Autodesk Inventor part; units mm, degrees
ref_plane "YZ Plane" through (0, 0, 0) normal (1, 0, 0) x (0, 1, 0)
ref_plane "XZ Plane" through (0, 0, 0) normal (0, 1, 0) x (-1, 0, 0)
ref_plane "XY Plane" through (0, 0, 0) normal (0, 0, 1) x (1, 0, 0)
sketch "Sketch1" plane through (0, 0, 0) normal (0, 0, 1) x (1, 0, 0)
  line L0 (-53.34, 0) -> (53.34, 0)
  line L1 (0, -7.0485) -> (0, 42.291)
  line L2 (-38.1, 0) -> (38.1, 0)
  arc A0 (16.1925, 19.05) -> (-16.1925, 19.05) centre (0, 19.05) ccw
  line L3 (-38.1, 6.35) -> (-22.5425, 6.35)
  line L4 (22.5425, 6.35) -> (38.1, 6.35)
  line L5 (38.1, 0) -> (38.1, 6.35)
  line L6 (-38.1, 0) -> (-38.1, 6.35)
  line L7 (-16.1925, 19.05) -> (-16.1925, 12.7)
  line L8 (16.1925, 19.05) -> (16.1925, 12.7)
  arc A1 (-22.5425, 6.35) -> (-16.1925, 12.7) centre (-22.5425, 12.7) ccw
  arc A2 (16.1925, 12.7) -> (22.5425, 6.35) centre (22.5425, 12.7) ccw
  point P0 (0, 0)
  point P1 (-10.0453, 6.35)
  point P2 (10.0453, 6.35)
  dimension "d0" = 76.2
  dimension "d1" = 32.385
  dimension "d4" = 6.35
  dimension "d5" = 19.05
  dimension "d6" = 6.35
extrude "Extrusion1" add sketch "Sketch1" along normal mid plane 12.7
sketch "Sketch2" plane through (0, 0, 6.35) normal (0, 0, 1) x (1, 0, 0)
  arc A0 (16.1925, 19.05) -> (-16.1925, 19.05) centre (0, 19.05) ccw
  circle A1 centre (0, 19.05) radius 14.3129
  point P0 (0, 0)
  dimension "d9" = 28.6258
extrude "Extrusion2" cut sketch "Sketch2" against normal blind 11.1125
sketch "Sketch3" plane through (0, 19.05, -4.7625) normal (0, 0, 1) x (1, 0, 0)
  circle A0 centre (0, 0) radius 14.3129
  circle A1 centre (0, 0) radius 7.9375
  point P0 (0, -19.05)
  dimension "d14" = 15.875
extrude "Extrusion3" cut sketch "Sketch3" against normal through all contours A1
sketch "Sketch4" plane through (-38.1, 6.35, 6.35) normal (0, 1, 0) x (1, 0, 0)
  line L0 (15.5575, 12.7) -> (0, 12.7)
  arc A0 (5.3975, 9.7282) -> (5.3975, 2.9718) centre (5.3975, 6.35) ccw
  line L1 (-15.24, 6.35) -> (91.44, 6.35)
  line L2 (38.1, 15.24) -> (38.1, -2.54)
  arc A1 (10.16, 2.9718) -> (10.16, 9.7282) centre (10.16, 6.35) ccw
  line L3 (10.16, 9.7282) -> (5.3975, 9.7282)
  line L4 (10.16, 2.9718) -> (5.3975, 2.9718)
  line L5 (7.7788, 2.9718) -> (7.7788, 9.7282) construction
  point P0 (38.1, 6.35)
  point P1 (7.7788, 12.7)
  dimension "d16" = 3.3782
  dimension "d17" = 4.7625
extrude "Mount Slot" cut sketch "Sketch4" against normal through all
mirror "Mirror1" about plane through (0, 0, 0) normal (1, 0, 0) of "Mount Slot"
properties part number "side mount bearing block"
Part model, mm, in its own coordinate system. A direction names the side the tool comes from. Coordinates: 2 decimals unless noted, no trailing zeros. Loops run counter-clockwise (first coordinate to the right, second up) from the corner with the lowest first, then second, coordinate; pieces in that order, holes last. Notation, with made-up numbers: (-32.5, 58) - (-9.5, 58) arc R33 ccw to (-9.5, 97) - close; hole circle Ø6 at (87, 68.5). An arc over 180 degrees is marked (long way). Write item = value, one per line. Start each with the question number.
Item 1: Flat gauge pins, fed straight in: pin 1 Ø2 at (y, z) = (15, 3.5) entering from -X; pin 2 Ø1 at (x, z) = (21, 4) entering from +Y; pin 3 Ø7 at (y, z) = (14.5, 2) entering from +X. Where does each tip first touch, or does it go through?
Item 2: Cut at B-B, the plane x = 0. Give the cut face in (y, z), and give its area (3 significant figures).
Item 3: Cut at D-D, the plane x = -13.5. Give the cut face in (y, z), and give its area (3 significant figures).
Item 4: 3-axis set-ups, long thin cutter, end or side, ignore diameter. For faces 1 (the flat face through (6, 13, -4.762)), 2 (the flat face through (30, 6.35, -4)), 3 (the flat face through (-30, 6.35, -4)), 4 (the flat face through (-30, 3, 3.378)): which of +Z, -Z, +X, -X, +Y, -Y reach the whole face in a straight line?
Item 5: Cut at C-C, the plane y = 21. Give the cut face in (x, z).
Item 6: Cut at A-A, the plane z = 0. State how many separate pieces and enclosed holes the cut face has, and give its area (3 significant figures).
Item 7: Wall check: L1, parallel to Y at x = 0, z = 4; L2, parallel to Y at x = 0, z = -5.45; L3, parallel to X at y = 19, z = 2. Give the ranges that are in metal, low to high. Write a range as from..to.
Item 8: Mould opens along Z. For faces 5 (the cylindrical face through (-0.36, 35.24, -0.09)), 6 (the cylindrical face through (-36.08, 3.22, -0.07)), 7 (the flat face through (0, 3, 6.35)), 8 (the flat face through (-30, 3, -3.378)) say: released by +Z, released by -Z, zero draft, split by the parting line, or undercut.
The answers:
q1.pin_1 = -16.19
q1.pin_2 = 6.69
q1.pin_3 = 16.42
q2.outline = (0, -6.35) - (11.11, -6.35) - (11.11, -4.76) - (4.74, -4.76) - (4.74, 6.35) - (0, 6.35) - close; (26.99, -6.35) - (35.24, -6.35) - (35.24, 6.35) - (33.36, 6.35) - (33.36, -4.76) - (26.99, -4.76) - close
q2.area = 104 mm2
q3.outline = (0, -6.35) - (27.99, -6.35) - (27.99, 6.35) - (23.8, 6.35) - (23.8, -4.76) - (14.3, -4.76) - (14.3, 6.35) - (0, 6.35) - close
q3.area = 250 mm2
q4.face_1 = +Z
q4.face_2 = +Z, -Z, +X, +Y
q4.face_3 = +Z, -Z, -X, +Y
q4.face_4 = +Y, -Y
q5.outline = (-16.07, -6.35) - (-7.69, -6.35) - (-7.69, -4.76) - (-14.18, -4.76) - (-14.18, 6.35) - (-16.07, 6.35) - close; (7.69, -6.35) - (16.07, -6.35) - (16.07, 6.35) - (14.18, 6.35) - (14.18, -4.76) - (7.69, -4.76) - close
q6.separate_pieces = 3
q6.enclosed_holes = 1
q6.area = 534 mm2
q7.L1 = 0..4.74, 33.36..35.24
q7.L2 = 0..11.11, 26.99..35.24
q7.L3 = -16.19..-14.31, 14.31..16.19
q8.face_5 = zero draft
q8.face_6 = undercut
q8.face_7 = released by +Z
q8.face_8 = undercut
